Can you work these out from the model? Positions are in its coordinate system, mm. Face numbers are marked on the shaded views. A direction names the side the tool comes from. Round coordinates to 2 decimals unless told otherwise and drop trailing zeros. Order: outer loops, then holes, each group sorted by start corner. A loop starts at its lowest first (then second) coordinate and runs counter-clockwise, first axis right, second up.
Q1. Will these pins go through, and if not, where does the flat tip stop? P1, Ø9, axis at x = -26, y = 70.5, coming from the -Z side; P2, Ø2, axis at x = -8.5, y = 5, coming from the -Z side; P3, Ø3, axis at x = -5, z = -9.5, coming from the +Y side.
Q2. If we section it at D-D (z = -32): Please give me the cut outline in (x, y), plus the area to 3 significant figures.
Q3. If we section it at C-C (x = -25.5): Please give me the cut outline in (y, z), plus the area to 3 significant figures.
Q4. We'd pull the mould along X, two halves only. Please class the marked faces 1, 2, 3 and 4: pulls with the +X half, pulls with the -X half, needs draft (parallel to the pull), parting line crosses it, or undercut.
Q5. If we section it at B-B (y = 30): Please give me the cut outline in (x, z), plus the area to 3 significant figures.
Q6. If we section it at A-A (x = -12): Please give me the cut outline in (y, z).
Q7. For the marked faces 5, 6 and 7, which set-ups out of +Z, -Z, +X, -X, +Y, -Y let a thin tool reach every point of the face, with its end or its side?
Q8. If I drill on line 1 (X direction, y = 9.5, z = -19); line 2 (X direction, y = 71.55, z = 1.4); line 3 (X direction, y = 71, z = -1), over which ranges is the centre line in solid material (lowest first)?
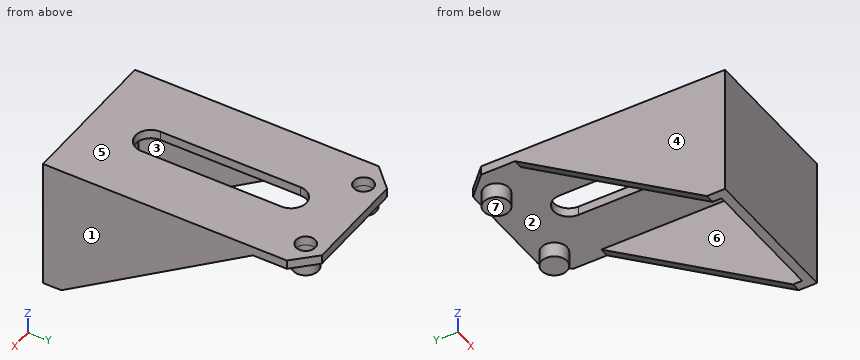
from build123d import *
from build123d.topology import SkipClean

# Parameters (mm, degrees)
SKETCH1_R                = 1.55
SKETCH1_R_2              = 1.5
SKETCH1_R_3              = 11
SKETCH1_R_4              = 3.175
BOSS_EXTRUDE1_DEPTH      = 3
BOSS_EXTRUDE2_START      = 3
SKETCH2_R                = 4.175
SKETCH2_R_2              = 3.175
BOSS_EXTRUDE2_DEPTH      = 3
BOSS_EXTRUDE3_START      = 2
SKETCH3_R                = 4.175
BOSS_EXTRUDE3_DEPTH      = 2
BOSS_EXTRUDE4_DEPTH      = 40
BOSS_EXTRUDE4_DEPTH_BACK = 3
SKETCH5_W                = 3
SKETCH5_H                = 5
BOSS_EXTRUDE5_DEPTH      = 3
BOSS_EXTRUDE7_DEPTH      = 3
BOSS_EXTRUDE9_DEPTH      = 3
BOSS_EXTRUDE10_START     = -3
SKETCH9_R                = 1.55
SKETCH9_R_2              = 1.5
SKETCH9_R_3              = 11
BOSS_EXTRUDE10_DEPTH     = 3
CUT_EXTRUDE1_DEPTH       = 3
SKETCH11_W               = 3
SKETCH11_H               = 75.55
BOSS_EXTRUDE11_DEPTH     = 3
CHAMFER1_SIZE            = 3
BOSS_EXTRUDE12_DEPTH     = 3
BOSS_EXTRUDE13_DEPTH     = 3
BOSS_EXTRUDE14_DEPTH     = 3


with BuildPart() as part:
    # Sketch1 → Boss-Extrude1 (new body)
    with BuildSketch(Plane.XY):
        Polygon((-33.421286346, -6), (-33.421286346, 36.5), (-33.421286346, 72.55), (-28.421286346, 77.55), (4.078713654, 77.55), (9.078713654, 72.55), (9.078713654, 36.5), (9.078713654, -6), align=None)
        with Locations((2.92772434, 30.5)):
            Circle(SKETCH1_R, mode=Mode.SUBTRACT)
        with Locations(Location((2.92772434, -0.5, 0), (0, 0, 180))):
            Circle(SKETCH1_R_2, mode=Mode.SUBTRACT)
        with Locations((-27.671286346, -0.5)):
            Circle(SKETCH1_R_2, mode=Mode.SUBTRACT)
        with Locations(Location((-28.07227566, 30.5, 0), (0, 0, 180))):
            Circle(SKETCH1_R_2, mode=Mode.SUBTRACT)
        with Locations((-12.171286346, 15.25)):
            Circle(SKETCH1_R_3, mode=Mode.SUBTRACT)
        with Locations((-27.421286346, 71.55)):
            Circle(SKETCH1_R_4, mode=Mode.SUBTRACT)
        with Locations(Location((3.078713654, 71.55, 0), (0, 0, 180))):
            Circle(SKETCH1_R_4, mode=Mode.SUBTRACT)
    extrude(amount=BOSS_EXTRUDE1_DEPTH)

    # Sketch2 → Boss-Extrude2 (add)
    # profile 1 of 2: a face of its own
    with SkipClean():  # the faces are left unmerged after this step: merging them gives an invalid solid
        with BuildSketch(Plane(origin=(0, 0, 0), x_dir=(-1, 0, 0), z_dir=(0, 0, -1)).offset(BOSS_EXTRUDE2_START)):
            with Locations((-3.078713654, 71.55)):
                Circle(SKETCH2_R)
            with Locations((-3.078713654, 71.55)):
                Circle(SKETCH2_R_2, mode=Mode.SUBTRACT)
        # profile 2 of 2: a face of its own
        with BuildSketch(Plane(origin=(0, 0, 0), x_dir=(-1, 0, 0), z_dir=(0, 0, -1)).offset(BOSS_EXTRUDE2_START)):
            with Locations((27.421286346, 71.55)):
                Circle(SKETCH2_R)
            with Locations((27.421286346, 71.55)):
                Circle(SKETCH2_R_2, mode=Mode.SUBTRACT)
        extrude(amount=-BOSS_EXTRUDE2_DEPTH)

    # Sketch3 → Boss-Extrude3 (add)
    with SkipClean():  # the faces are left unmerged after this step: merging them gives an invalid solid
        with BuildSketch(Plane(origin=(0, 0, -3), x_dir=(-1, 0, 0), z_dir=(0, 0, -1)).offset(BOSS_EXTRUDE3_START)):
            with Locations((-3.078713654, 71.55)):
                Circle(SKETCH3_R)
            with Locations((27.421286346, 71.55)):
                Circle(SKETCH3_R)
        extrude(amount=-BOSS_EXTRUDE3_DEPTH)

    # Sketch5 → Boss-Extrude5 (add)
    with SkipClean():  # the faces are left unmerged after this step: merging them gives an invalid solid
        with BuildSketch(Plane.XY.offset(3)):
            with Locations((10.578713654, 45.531399611)):
                Rectangle(SKETCH5_W, SKETCH5_H)
            with Locations((-34.921286346, 45.531399611)):
                Rectangle(SKETCH5_W, SKETCH5_H)
        extrude(amount=-BOSS_EXTRUDE5_DEPTH)



with BuildPart() as body_2:
    # Sketch4 → Boss-Extrude4 (new, two sides: drawn at the far end of the back side and taken through both)
    with BuildSketch(Plane(origin=(0, 0, 0), x_dir=(-1, 0, 0), z_dir=(0, 0, -1)).offset(-BOSS_EXTRUDE4_DEPTH_BACK)):
        Polygon((33.421286346, -6), (-9.078713654, -6), (-9.078713654, -3), (-12.078713654, -3), (-12.078713654, -9), (-9.078713654, -9), (34.421286346, -9), (36.421286346, -9), (36.421286346, -3), (33.421286346, -3), align=None)
    extrude(amount=BOSS_EXTRUDE4_DEPTH + BOSS_EXTRUDE4_DEPTH_BACK)


with BuildPart() as part_1:
    with SkipClean():  # the faces are left unmerged after this step: merging them gives an invalid solid
        add(part.part)

        add(body_2.part)  # Boss-Extrude7 merges body 2
        # Sketch6 → Boss-Extrude7 (add)
        with BuildSketch(Plane(origin=(9.078713654, 0, 0), x_dir=(0, 0, -1), z_dir=(1, 0, 0))):
            Polygon((0, 48.031399611), (40, -3), (36.080844313, -3), (0, 43.031399611), align=None)
        extrude(amount=BOSS_EXTRUDE7_DEPTH)

    # Sketch8 → Boss-Extrude9 (add)
    with SkipClean():  # the faces are left unmerged after this step: merging them gives an invalid solid
        with BuildSketch(Plane.ZY.offset(36.421286346)):
            Polygon((0, 48.031399611), (0, 43.031399611), (-36.080844313, -3), (-40, -3), align=None)
        extrude(amount=-BOSS_EXTRUDE9_DEPTH)

    # Sketch9 → Boss-Extrude10 (add)
    with SkipClean():  # the faces are left unmerged after this step: merging them gives an invalid solid
        with BuildSketch(Plane.XY.offset(3).offset(BOSS_EXTRUDE10_START)):
            with Locations((2.92772434, 30.5)):
                Circle(SKETCH9_R)
            with Locations((-28.07227566, 30.5)):
                Circle(SKETCH9_R_2)
            with Locations((-27.671286346, -0.5)):
                Circle(SKETCH9_R_2)
            with Locations((2.92772434, -0.5)):
                Circle(SKETCH9_R_2)
            with Locations((-12.171286346, 15.25)):
                Circle(SKETCH9_R_3)
        extrude(amount=BOSS_EXTRUDE10_DEPTH)

    # Sketch10 → Cut-Extrude1 (cut)
    with BuildSketch(Plane.XY.offset(3)):
        with BuildLine():
            Line((-7.171286346, 57.275), (-7.171286346, 11.275))
            ThreePointArc((-7.171286346, 11.275), (-12.171286346, 6.275), (-17.171286346, 11.275))
            Line((-17.171286346, 11.275), (-17.171286346, 57.275))
            ThreePointArc((-17.171286346, 57.275), (-12.171286346, 62.275), (-7.171286346, 57.275))
        make_face()
    extrude(amount=-CUT_EXTRUDE1_DEPTH, mode=Mode.SUBTRACT)

    # Sketch11 → Boss-Extrude11 (add)
    with BuildSketch(Plane.XY.offset(3)):
        with Locations((-34.921286346, 34.775)):
            Rectangle(SKETCH11_W, SKETCH11_H)
        with Locations((10.578713654, 34.775)):
            Rectangle(SKETCH11_W, SKETCH11_H)
    extrude(amount=-BOSS_EXTRUDE11_DEPTH)

    # Chamfer1
    chamfer1_edges = [part_1.edges().sort_by_distance(p)[0] for p in [
        (-36.421286346, 72.55, 1.5),
        (12.078713654, 72.55, 1.5),
    ]]
    chamfer(chamfer1_edges, length=CHAMFER1_SIZE - 0.0001)  # a hair under: the kernel refuses the full size

    # Sketch12 → Boss-Extrude12 (add)
    with BuildSketch(Plane(origin=(12.078713654, 0, 0), x_dir=(0, 0, -1), z_dir=(1, 0, 0))):
        Polygon((-3, 64.55), (-3, -9), (40, -9), (40, -3), align=None)
    extrude(amount=-BOSS_EXTRUDE12_DEPTH)

    # Sketch13 → Boss-Extrude13 (add)
    with BuildSketch(Plane.ZY.offset(36.421286346)):
        Polygon((3, -9), (3, 64.55), (-40, -3), (-40, -9), align=None)
    extrude(amount=-BOSS_EXTRUDE13_DEPTH)

    # Sketch14 → Boss-Extrude14 (add)
    with BuildSketch(Plane.XY.offset(3)):
        Polygon((-36.421286346, 70.964213562), (-36.421286346, 69.55), (-28.421286346, 77.55), (4.078713654, 77.55), (12.078713654, 69.55), (12.078713654, 70.964213562), (4.992927216, 78.05), (-29.335499908, 78.05), align=None)
    extrude(amount=-BOSS_EXTRUDE14_DEPTH)


solid = part_1.part
Solution:
1. P1: stops at z = -5
1. P2: stops at z = 0
1. P3: stops at y = -6
2. outline: (-36.42, -9) - (12.08, -9) - (12.08, 9.57) - (9.08, 9.57) - (9.08, -6) - (-33.42, -6) - (-33.42, 9.57) - (-36.42, 9.57) - close
2. area: 239 mm2
3. outline: (-9, -40) - (-6, -40) - (-6, 0) - (67.84, 0) - (67.84, -5) - (75.26, -5) - (75.26, 0) - (78.05, 0) - (78.05, 3) - (74.08, 3) - (74.08, -3) - (69.02, -3) - (69.02, 3) - (-9, 3) - close
3. area: 388 mm2
4. face 1: pulls with the +X half
4. face 2: undercut
4. face 3: undercut
4. face 4: pulls with the -X half
5. outline: (-36.42, -18.99) - (-33.42, -18.99) - (-33.42, 0) - (-17.17, 0) - (-17.17, 3) - (-36.42, 3) - close; (-7.17, 0) - (9.08, 0) - (9.08, -18.99) - (12.08, -18.99) - (12.08, 3) - (-7.17, 3) - close
5. area: 229 mm2
6. outline: (-9, -40) - (-6, -40) - (-6, 0) - (6.28, 0) - (6.28, 3) - (-9, 3) - close; (62.27, 0) - (78.05, 0) - (78.05, 3) - (62.27, 3) - close
7. face 5: +Z, +X, -X, +Y, -Y
7. face 6: -Z, +Y
7. face 7: -Z, +X, -X, +Y
8. line 1: x = -36.42 to -33.42, 9.08 to 12.08
8. line 2: x = -35.84 to -30.6, -24.25 to -0.1, 6.25 to 11.49
8. line 3: x = -31.56 to -30.55, -24.29 to -23.28, -1.06 to -0.05, 6.21 to 7.22
